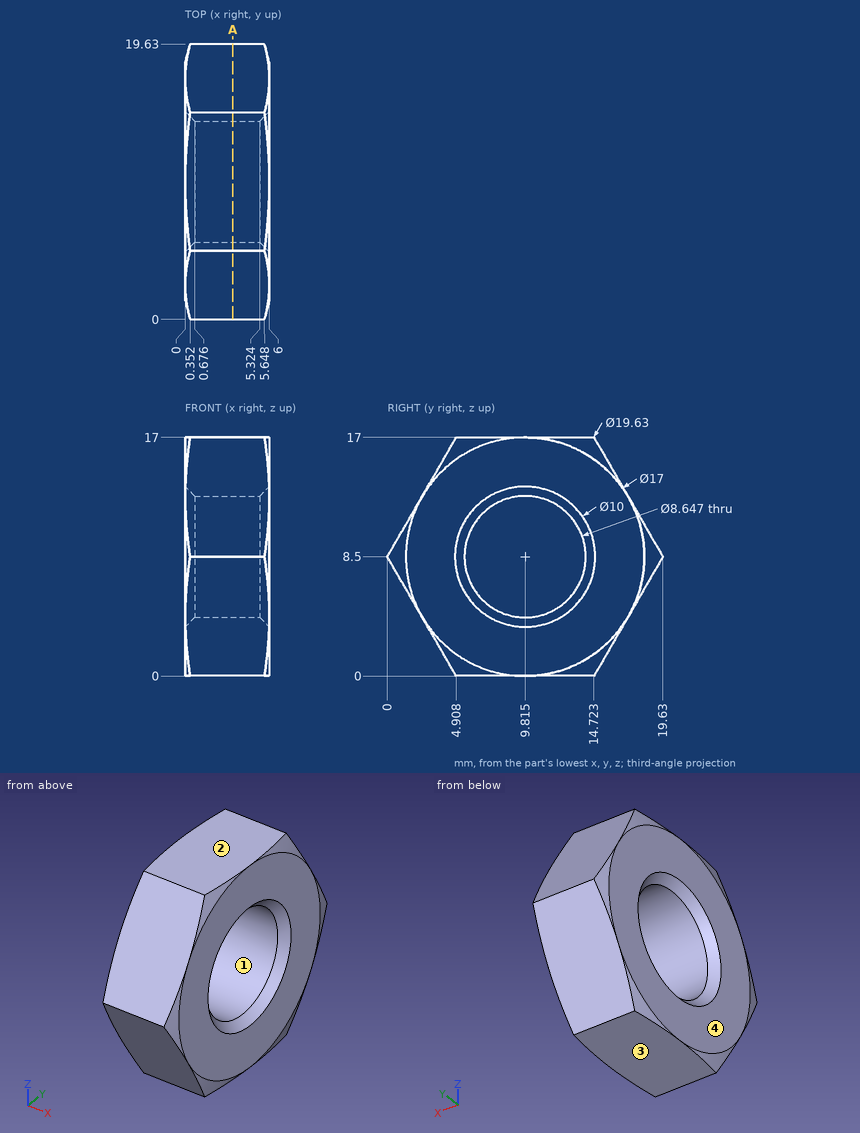
Source: three-view drawing plus pictorial views. Frame: mm from the lowest corner of the part. Round coordinates to 2 decimals unless told otherwise and drop trailing zeros. Loops run counter-clockwise (first coordinate to the right, second up) from the corner with the lowest first, then second, coordinate; pieces in that order, holes last. Notation, with made-up numbers: M 6.5,37.5 L 55.5,37.5 A26 cw 55.5,67.5 Z; hole C 1.25,79 d9. An arc over 180 degrees is marked long. Put each result on its own line as item: value. Start each with the question number.
(1) Material intervals for line 1 along Y through (x, z) = (3.3, 7.5); line 2 along Y through (x, z) = (2.75, 7) (1 decimal); line 3 along Z through (x, y) = (1.8, 11), sorted ascending. Write a range as [from, to].
(2) Section query A-A (x = 3.4). Return loops of the section in (y, z) (1 decimal).
(3) Draft query along Z for the marked faces 1, 2, 3 and 4. Return one class per face: +Z half, -Z half, draft (parallel to the pull), parting line (faces both ways), or undercut.
(4) Contact query for a flat-ended pin moving along its axis: pin 1 Ø1.5 at (x, z) = (1, 9) entering from -Y. Output: stop coordinate, or through.
Findings below:
1. line 1: y = [0.58, 5.61], [14.02, 19.05]
1. line 2: y = [0.9, 5.8], [13.9, 18.8]
1. line 3: z = [0, 4.34], [12.66, 17]
2. outline: M 0,8.5 L 4.9,0 L 14.7,0 L 19.6,8.5 L 14.7,17 L 4.9,17 Z; hole C 9.8,8.5 d8.6
3. face 1: undercut
3. face 2: +Z half
3. face 3: -Z half
3. face 4: draft
4. pin 1: stops at y = 0
